```python
from build123d import *

# Parameters (mm, degrees)
SKETCH2_W           = 20
SKETCH2_H           = 200
BOSS_EXTRUDE1_DEPTH = 5
BOSS_EXTRUDE2_DEPTH = 3
LPATTERN1_COUNT     = 33
LPATTERN1_PITCH     = 6


with BuildPart() as part:
    # Sketch2 → Boss-Extrude1 (new body)
    with BuildSketch(Plane(origin=(0, 0, 0), x_dir=(1, 0, 0), z_dir=(0, 1, 0))):
        Rectangle(SKETCH2_W, SKETCH2_H)
    extrude(amount=BOSS_EXTRUDE1_DEPTH)

    # Sketch3 → Boss-Extrude2 (add)
    with BuildSketch(Plane(origin=(0, 5, 0), x_dir=(1, 0, 0), z_dir=(0, 1, 0))):
        Polygon((-10, -100), (0, -98.236730193), (10, -100), (10, -97), (0, -95.236730193), (-10, -97), align=None)
    boss_extrude2 = extrude(amount=BOSS_EXTRUDE2_DEPTH)

    # LPattern1: Boss-Extrude2 ×33
    with Locations(*[(0, 0, -i * LPATTERN1_PITCH) for i in range(1, LPATTERN1_COUNT)]):
        add(boss_extrude2)


solid = part.part
```
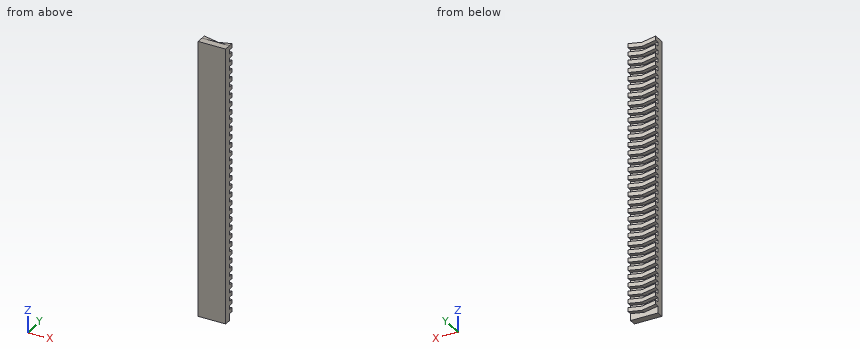
Model file for the job. Use its own axes, mm. Coordinates: 2 decimals unless noted, no trailing zeros. One line per question, with ' | ' between items. Start each with the question number.
Q1. Cut at A-A, the plane y = 6.5. Give the number of separate pieces and of enclosed holes in the cut face, then the cut area to 3 significant figures.
Q2. Pin check, flat tip, straight feed: pin 1 (1.4 mm diameter, centred on x = -2, z = 87.5, fed in from +Y). Stop position of the tip, or through.
Q3. Drill centre line: line 1 (Y direction, x = 7.5, z = 72). Where is it in solid material? Low to high. Write a range as [from, to].
Answer below:
1) separate pieces: 33 | enclosed holes: 0 | area: 1,980 mm^2
2) pin 1: y = 5
3) line 1: [0, 5]
